Build history of the part. All positions in model axes, mm. A direction names the side the tool comes from. Give positions to 0.01 mm unless a question says otherwise; leave off trailing zeros. Order: outer loops, then holes, each group sorted by start corner. A loop starts at its lowest first (then second) coordinate and runs counter-clockwise, first axis right, second up. Notation, with made-up numbers: (85, -1) - (134, -1) arc R17 ccw to (134, 20) - close; hole circle Ø9 at (20.25, -14). An arc over 180 degrees is marked (long way). Use a Markdown table: item, result.
Autodesk Inventor part; units mm, degrees
ref_plane "YZ Plane" through (0, 0, 0) normal (1, 0, 0) x (0, 1, 0)
ref_plane "XZ Plane" through (0, 0, 0) normal (0, 1, 0) x (-1, 0, 0)
ref_plane "XY Plane" through (0, 0, 0) normal (0, 0, 1) x (1, 0, 0)
sketch "Sketch1" plane through (0, 0, 0) normal (0, 0, 1) x (1, 0, 0)
  line L0 (-40, 15) -> (40, 15)
  line L1 (40, 15) -> (40, -15)
  line L2 (40, -15) -> (-40, -15)
  line L3 (-40, -15) -> (-40, 15)
  line L4 (-40, 15) -> (40, -15) construction
  line L5 (40, 15) -> (-40, -15) construction
  point P0 (0, 0)
  dimension "d0" = 80
  dimension "d1" = 30
extrude "Extrusion1" add sketch "Sketch1" along normal mid plane 3
sketch "Sketch3" plane through (0, 0, 1.5) normal (0, 0, 1) x (1, 0, 0)
  line L0 (23.5315, 18) -> (23.5315, 15)
  line L1 (-23.4685, 18) -> (-23.4685, 15)
  line L2 (-23.4685, 15) -> (23.5315, 15)
  line L3 (23.5315, 15) -> (23.5315, 12)
  line L4 (23.5315, 12) -> (-23.4685, 12)
  line L5 (-23.4685, 12) -> (-23.4685, 15)
  line L6 (-40, 15) -> (-40, -15)
  line L7 (-40, 5) -> (-37, 5)
  line L8 (-37, 5) -> (-37, -5)
  line L9 (-37, -5) -> (-40, -5)
  line L10 (-40, -5) -> (-40, 5)
  line L11 (40, -15) -> (40, 15)
  line L12 (40, -5) -> (37, -5)
  line L13 (37, -5) -> (37, 5)
  line L14 (37, 5) -> (40, 5)
  line L15 (40, 5) -> (40, -5)
  line L16 (-40, -15) -> (40, -15)
  line L17 (40, 15) -> (-40, 15)
  line L18 (-23.4685, -15) -> (23.5315, -15)
  line L19 (23.5315, -15) -> (23.5315, -12)
  line L20 (23.5315, -12) -> (-23.4685, -12)
  line L21 (-23.4685, -12) -> (-23.4685, -15)
  line L22 (-14.9948, 8) -> (-11.9948, 8)
  line L23 (-11.9948, 8) -> (-11.9948, -8)
  line L24 (-11.9948, -8) -> (-14.9948, -8)
  line L25 (-14.9948, -8) -> (-14.9948, 8)
  line L26 (1.5, 8) -> (1.5, -8)
  line L27 (1.5, -8) -> (-1.5, -8)
  line L28 (-1.5, -8) -> (-1.5, 8)
  line L29 (-1.5, 8) -> (1.5, 8)
  line L30 (12.0052, 8) -> (15.0052, 8)
  line L31 (15.0052, 8) -> (15.0052, -8)
  line L32 (15.0052, -8) -> (12.0052, -8)
  line L33 (12.0052, -8) -> (12.0052, 8)
  dimension "d27" = 3
  dimension "d28" = 3
  dimension "d29" = 3
  dimension "d30" = 30
  dimension "d31" = 10
  dimension "d32" = 10
  dimension "d41" = 3
extrude "Extrusion3" cut sketch "Sketch3" against normal blind 3 contours L2 L3 L4 L5 | L7 L8 L9 L6 | L11 L12 L13 L14 | L21 L20 L19 L16 | L22 L23 L24 L25 | L26 L27 L28 L29 | L30 L31 L32 L33
equation "\"d31\" = 0.333333 * d30"
equation "\"d32\" = d31"
properties part number "Camera-Holder_Bearing-Side"
1) Slice it at C-C (y = -0.5). Write the cut outline in (x, z), and give its area (3 significant figures).
Computed:
| item | result |
|---|---|
| outline | (-37, -1.5) - (-14.99, -1.5) - (-14.99, 1.5) - (-37, 1.5) - close; (-11.99, -1.5) - (-1.5, -1.5) - (-1.5, 1.5) - (-11.99, 1.5) - close; (1.5, -1.5) - (12.01, -1.5) - (12.01, 1.5) - (1.5, 1.5) - close; (15.01, -1.5) - (37, -1.5) - (37, 1.5) - (15.01, 1.5) - close |
| area | 195 mm² |
2) Slice it at B-B (z = -0.3). State how many separate pieces and enclosed holes the cut face has, and give its area (3 significant figures).
Computed:
| item | result |
|---|---|
| separate pieces | 1 |
| enclosed holes | 3 |
| area | 1,910 mm² |
3) Slice it at A-A (y = 6). Write the cut outline in (x, z).
Computed:
| item | result |
|---|---|
| outline | (-40, -1.5) - (-14.99, -1.5) - (-14.99, 1.5) - (-40, 1.5) - close; (-11.99, -1.5) - (-1.5, -1.5) - (-1.5, 1.5) - (-11.99, 1.5) - close; (1.5, -1.5) - (12.01, -1.5) - (12.01, 1.5) - (1.5, 1.5) - close; (15.01, -1.5) - (40, -1.5) - (40, 1.5) - (15.01, 1.5) - close |
4) Tool access for faces 1 (the flat face through (-23.468, -13, 0)), 2 (the flat face through (-14.995, 0, 0)), 3 (the flat face through (39, -5, 0)): list every direction of +Z, -Z, +X, -X, +Y, -Y with a clear straight run to the whole face (end or side of a thin tool).
Computed:
| item | result |
|---|---|
| face 1 | +Z, -Z, -Y |
| face 2 | +Z, -Z |
| face 3 | +Z, -Z, +X |
5) Wall check: line 1 (X direction, y = -7.25, z = -0.85); line 2 (X direction, y = 3.75, z = 1.15); line 3 (Y direction, x = -12.5, z = 0.85). Give the ranges that are in metal, low to high. Write a range as from..to.
Computed:
| item | result |
|---|---|
| line 1 | x = -40..-14.99, -11.99..-1.5, 1.5..12.01, 15.01..40 |
| line 2 | x = -37..-14.99, -11.99..-1.5, 1.5..12.01, 15.01..37 |
| line 3 | y = -12..-8, 8..12 |
6) Slice it at D-D (x = -16). Write the cut outline in (y, z), and give its area (3 significant figures).
Computed:
| item | result |
|---|---|
| outline | (-12, -1.5) - (12, -1.5) - (12, 1.5) - (-12, 1.5) - close |
| area | 72.0 mm² |
7) Pin check, flat tips, straight feed: P1, Ø1.5, axis at x = 12, z = 0, coming from the +Y side; P2, Ø1, axis at x = -8.5, z = -0.5, coming from the -Y side; P3, Ø0.9, axis at y = -1, z = 0.5, coming from the +X side. Stop position of each tip, or through.
Computed:
| item | result |
|---|---|
| P1 | stops at y = 12 |
| P2 | stops at y = -12 |
| P3 | stops at x = 37 |
